Autodesk Inventor part; units mm, degrees
ref_plane "YZ Plane" through (0, 0, 0) normal (1, 0, 0) x (0, 1, 0)
ref_plane "XZ Plane" through (0, 0, 0) normal (0, 1, 0) x (-1, 0, 0)
ref_plane "XY Plane" through (0, 0, 0) normal (0, 0, 1) x (1, 0, 0)
sketch "Sketch1" plane through (0, 0, 0) normal (0, 1, 0) x (-1, 0, 0)
  circle A0 centre (0, 0) radius 1.778
  dimension "d0" = 3.556
extrude "Extrusion1" add sketch "Sketch1" along normal blind 25.4
sketch "Sketch3" plane through (0, 25.4, 0) normal (0, 1, 0) x (1, 0, 0)
  circle A0 centre (0, 0) radius 3.81
  dimension "d4" = 7.62
extrude "Extrusion2" add sketch "Sketch3" along normal blind 2.032
fillet "Fillet1" radius 3.175 1 edges at (-3.81, 27.432, 0)
properties part number "screw_o.15"
Build history of the part. All positions in model axes, mm. A direction names the side the tool comes from. Round coordinates to 2 decimals unless told otherwise and drop trailing zeros. Write each loop counter-clockwise with the first axis right and the second up, starting at its lowest first coordinate (ties: lowest second). Pieces come first, ordered by that corner, then holes. Notation, with made-up numbers: (66.5, 35.5) -> (83.5, 35.5) arc R25 cw to (83.5, 52.5) -> close; hole circle Ø3 at (66.5, 19). An arc over 180 degrees is marked (long way). Put each result on its own line as item: value.
Item 1: Tool access for faces 1 (the face through (0, 27.432, 0)), 2 (the face through (2, 25.4, 1)): list every direction of +Z, -Z, +X, -X, +Y, -Y with a clear straight run to the whole face (end or side of a thin tool).
Here are the results:
face 1: +Z, -Z, +X, -X, +Y
face 2: -Y
Item 2: Wall check: probe 1 along Y at (x, z) = (0, 1); probe 2 along Y at (x, z) = (-0.5, -2.5); probe 3 along X at (y, z) = (19, -1). Give the ranges that are in metal, low to high. Write a range as from..to.
Here are the results:
probe 1: y = 0..27.43
probe 2: y = 25.4..26.94
probe 3: x = -1.47..1.47
Item 3: Flat gauge pins, fed straight in: P1, Ø1.5, axis at x = 0, z = -2, coming from the +Y side; P2, Ø1.5, axis at y = 11.5, z = -1, coming from the +X side. Where does each tip first touch, or does it go through?
Here are the results:
P1: stops at y = 27.41
P2: stops at x = 1.76
Item 4: Slice it at A-A, the plane y = 3.5. Give the cut face in (x, z).
Here are the results:
outline: circle Ø3.56 at (0, 0)
